The model under review builds one solid part; all positions refer to its coordinate system, in mm. Round coordinates to 2 decimals unless told otherwise and drop trailing zeros. Order: outer loops, then holes, each group sorted by start corner. A loop starts at its lowest first (then second) coordinate and runs counter-clockwise, first axis right, second up. Notation, with made-up numbers: (-0.75, -0.75) -> (44.25, -0.75) arc R15 ccw to (44.25, 28.25) -> close; hole circle Ø4 at (0, 62). An arc over 180 degrees is marked (long way). Return JSON: item names as keys, results as strings. Group by question number.
from build123d import *

# Parameters (mm, degrees)
BASE_FLANGE1_DEPTH = 6
HEM1_START         = -50
HEM1_DEPTH         = 100
HEM1_START_2       = -150
HEM1_2_DEPTH       = 50
HEM1_START_3       = 100
HEM1_3_DEPTH       = 50
SKETCH14_R         = 15
CUT_EXTRUDE1_DEPTH = 10


# Read off the part's stored shape, not the designer's step: Hem1
# Sheet-metal steps are written as plain solids
with BuildPart() as part:
    # Sketch1 → Base-Flange1 (new body)
    with BuildSketch(Plane.XY):
        with BuildLine():
            Line((100, 75), (50, 75))
            Line((50, 75), (50, 115))
            Line((50, 115), (-50, 115))
            Line((-50, 115), (-50, 75))
            Line((-50, 75), (-100, 75))
            Line((-100, 75), (-100, 115))
            Line((-100, 115), (-150, 115))
            Line((-150, 115), (-150, 20))
            ThreePointArc((-150, 20), (-144.142135624, 5.857864376), (-130, 0))
            Line((-130, 0), (130, 0))
            ThreePointArc((130, 0), (144.142135624, 5.857864376), (150, 20))
            Line((150, 20), (150, 115))
            Line((150, 115), (100, 115))
            Line((100, 115), (100, 75))
        make_face()
    extrude(amount=-BASE_FLANGE1_DEPTH)

    # Hem1 outline → Hem1 (add)
    with BuildSketch(Plane.YZ.offset(HEM1_START)):
        with BuildLine():
            Line((84.284293607, 5.39157987), (87.101122984, 0.093894313))
            Line((87.101122984, 0.093894313), (111.71369906, 13.18063315))
            ThreePointArc((111.71369906, 13.18063315), (121.792070084, 8.69345327), (115, 0))
            Line((115, 0), (115, -6))
            ThreePointArc((115, -6), (127.613844442, 10.144984643), (108.896869684, 18.478318707))
            Line((108.896869684, 18.478318707), (84.284293607, 5.39157987))
        make_face()
    extrude(amount=HEM1_DEPTH)

    # Hem1 2 outline → Hem1 2 (add)
    with BuildSketch(Plane.YZ.offset(HEM1_START_2)):
        with BuildLine():
            Line((84.284293607, 5.39157987), (87.101122984, 0.093894313))
            Line((87.101122984, 0.093894313), (111.71369906, 13.18063315))
            ThreePointArc((111.71369906, 13.18063315), (121.792070084, 8.69345327), (115, 0))
            Line((115, 0), (115, -6))
            ThreePointArc((115, -6), (127.613844442, 10.144984643), (108.896869684, 18.478318707))
            Line((108.896869684, 18.478318707), (84.284293607, 5.39157987))
        make_face()
    extrude(amount=HEM1_2_DEPTH)

    # Hem1 3 outline → Hem1 3 (add)
    with BuildSketch(Plane.YZ.offset(HEM1_START_3)):
        with BuildLine():
            Line((84.284293607, 5.39157987), (87.101122984, 0.093894313))
            Line((87.101122984, 0.093894313), (111.71369906, 13.18063315))
            ThreePointArc((111.71369906, 13.18063315), (121.792070084, 8.69345327), (115, 0))
            Line((115, 0), (115, -6))
            ThreePointArc((115, -6), (127.613844442, 10.144984643), (108.896869684, 18.478318707))
            Line((108.896869684, 18.478318707), (84.284293607, 5.39157987))
        make_face()
    extrude(amount=HEM1_3_DEPTH)

    # Sketch14 → Cut-Extrude1 (cut)
    with BuildSketch(Plane.XY):
        with Locations((100, 40)):
            Circle(SKETCH14_R)
        with Locations((0, 40)):
            Circle(SKETCH14_R)
        with Locations((-100, 40)):
            Circle(SKETCH14_R)
    extrude(amount=-CUT_EXTRUDE1_DEPTH, mode=Mode.SUBTRACT)


solid = part.part
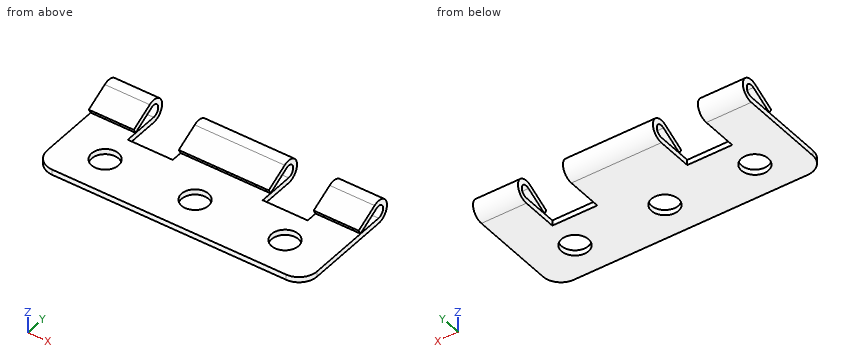
Item 1: Consider section D-D on z = 2.75. State the section outline as (x, y) points, plus the area to 3 significant figures.
Item 2: Consider section A-A on y = 40. State the section outline as (x, z) points, plus the area to 3 significant figures.
Item 3: Consider section C-C on y = 94.5. State the section outline as (x, z) points.
Item 4: Insertion check: pin 1 Ø3 at (x, z) = (17.5, 3.5) entering from +Y; pin 2 Ø3 at (x, z) = (-6.5, 15) entering from -Y; pin 3 Ø12 at (x, z) = (8.5, 14.5) entering from +Y. Each pin has a flat end and moves straight along its axis. Give the tip position at first contact, or say it passes through.
Item 5: Wall thickness on line 1 along X through (y, z) = (106, 13.5); line 2 along Z through (x, y) = (5, 115); line 3 along Y through (x, z) = (-77.5, -1.25): over which ranges is each line inside the solid? List them lowest first.
Item 6: Consider section B-B on x = -33.5. State the section outline as (y, z) points.
Values:
{
 "1": {"outline": "(-150, 85.69) -> (-100, 85.69) -> (-100, 92.1) -> (-150, 92.1) -> close; (-150, 120.56) -> (-100, 120.56) -> (-100, 127.29) -> (-150, 127.29) -> close; (-50, 85.69) -> (50, 85.69) -> (50, 92.1) -> (-50, 92.1) -> close; (-50, 120.56) -> (50, 120.56) -> (50, 127.29) -> (-50, 127.29) -> close; (100, 85.69) -> (150, 85.69) -> (150, 92.1) -> (100, 92.1) -> close; (100, 120.56) -> (150, 120.56) -> (150, 127.29) -> (100, 127.29) -> close", "area": "2,630 mm^2"},
 "2": {"outline": "(-150, -6) -> (-115, -6) -> (-115, 0) -> (-150, 0) -> close; (-85, -6) -> (-15, -6) -> (-15, 0) -> (-85, 0) -> close; (15, -6) -> (85, -6) -> (85, 0) -> (15, 0) -> close; (115, -6) -> (150, -6) -> (150, 0) -> (115, 0) -> close", "area": "1,260 mm^2"},
 "3": {"outline": "(-150, -6) -> (-100, -6) -> (-100, 0) -> (-150, 0) -> close; (-150, 4.03) -> (-100, 4.03) -> (-100, 10.82) -> (-150, 10.82) -> close; (-50, -6) -> (50, -6) -> (50, 0) -> (-50, 0) -> close; (-50, 4.03) -> (50, 4.03) -> (50, 10.82) -> (-50, 10.82) -> close; (100, -6) -> (150, -6) -> (150, 0) -> (100, 0) -> close; (100, 4.03) -> (150, 4.03) -> (150, 10.82) -> (100, 10.82) -> close"},
 "4": {"pin 1": "y = 127.85", "pin 2": "y = 99.53", "pin 3": "y = 127.91"},
 "5": {"line 1": "-150 to -100, -50 to 50, 100 to 150", "line 2": "-6 to 0, 14 to 20", "line 3": "0 to 75"},
 "6": {"outline": "(0, -6) -> (115, -6) arc R13 ccw (long way) to (108.9, 18.48) -> (84.28, 5.39) -> (87.1, 0.09) -> (111.71, 13.18) arc R7 cw (long way) to (115, 0) -> (0, 0) -> close"}
}
